Autodesk Inventor part; units mm, degrees
ref_plane "YZ Plane" through (0, 0, 0) normal (1, 0, 0) x (0, 1, 0)
ref_plane "XZ Plane" through (0, 0, 0) normal (0, 1, 0) x (-1, 0, 0)
ref_plane "XY Plane" through (0, 0, 0) normal (0, 0, 1) x (1, 0, 0)
sketch "Sketch1" plane through (0, 0, 0) normal (0, 0, 1) x (1, 0, 0)
  line L0 (-22, -22) -> (22, -22)
  line L1 (22, -22) -> (22, 22)
  line L2 (22, 22) -> (-22, 22)
  line L3 (-22, 22) -> (-22, -22)
  line L4 (-22, -22) -> (22, 22) construction
  line L5 (22, -22) -> (-22, 22) construction
  point P0 (0, 0)
  point P1 (0, 0)
  dimension "a" = 44
  dimension "d10" = 22
  dimension "d11" = 22
  dimension "d15" = 44
extrude "Extrusion1" add sketch "Sketch1" along normal blind 10
sketch "Sketch2" plane through (0, 0, 10) normal (0, 0, 1) x (1, 0, 0)
  circle A0 centre (0, 0) radius 18
  dimension "dg6" = 36
extrude "Extrusion2" add sketch "Sketch2" along normal blind 17
sketch "Sketch3" plane through (0, 0, 27) normal (0, 0, 1) x (1, 0, 0)
  circle A0 centre (0, 0) radius 18
  circle A1 centre (0, 0) radius 6
  dimension "d1" = 12
extrude "Extrusion3" cut sketch "Sketch3" against normal through all contours A1
chamfer "Chamfer1" distance 5 angle 45 4 edges at (22, 22, 5) (22, -22, 5) (-22, -22, 5) (-22, 22, 5)
sketch "Sketch4" plane through (0, 0, 0) normal (0, 0, -1) x (-1, 0, 0)
  circle A0 centre (0, 0) radius 6
  circle A1 centre (0, 0) radius 22 construction
  point P0 (17, 13.9642)
  point P1 (-17, -13.9642)
  point P2 (-17, 13.9642)
  point P3 (17, -13.9642)
  dimension "d16" = 44
  dimension "d17" = 34
hole "Hole1" at (-17, 13.9642, 0) at (17, -13.9642, 0) at (17, 13.9642, 0) at (-17, -13.9642, 0) direction (0, 0, 1) diameter 4.5 end through all
sketch "Sketch5" plane through (0, 0, 0) normal (0, 0, -1) x (-1, 0, 0)
  circle A0 centre (-17, 13.9642) radius 2.25
  circle A1 centre (17, 13.9642) radius 2.25
  circle A2 centre (-17, -13.9642) radius 2.25
  circle A3 centre (17, -13.9642) radius 2.25
hole "Hole2" at (17, 13.9642, 0) at (-17, 13.9642, 0) at (-17, -13.9642, 0) at (17, -13.9642, 0) direction (0, 0, 1) diameter 8 depth 4
equation "\"d15\" = a"
properties part number "fk12"
Verification items for the finished model (mm, model axes). A direction names the side the tool comes from. Coordinates: 2 decimals unless noted, no trailing zeros. Loops run counter-clockwise (first coordinate to the right, second up) from the corner with the lowest first, then second, coordinate; pieces in that order, holes last. Notation, with made-up numbers: (71, 37) -> (107, 37) arc R15 cw to (107, 46) -> close; hole circle Ø5 at (65, 73). An arc over 180 degrees is marked (long way). Answer in a Markdown table with one row per item.
1) Section check C-C (z = 17.5). Record the cut outline in (x, y).
The answers:
| item | result |
|---|---|
| outline | circle Ø36 at (0, 0); hole circle Ø12 at (0, 0) |
2) Access from +Z, -Z, +X, -X, +Y, -Y to the whole of each face (thin tool, end or side, straight path). Record for faces 1 (the face through (-15, -12, 4)), 2 (the face through (0, 20, 10)), 3 (the face through (-19, -20, 5)).
The answers:
| item | result |
|---|---|
| face 1 | -Z |
| face 2 | +Z |
| face 3 | +Z, -Z, -X, -Y |
3) Scan lines: line 1 along Y through (x, z) = (-17, 7); line 2 along Y through (x, z) = (-17, 1.25); line 3 along Y through (x, z) = (0, 18). Record each from-to range of solid material in increasing order. Write a range as from..to.
The answers:
| item | result |
|---|---|
| line 1 | y = -22..-16.21, -11.71..11.71, 16.21..22 |
| line 2 | y = -22..-17.96, -9.96..9.96, 17.96..22 |
| line 3 | y = -18..-6, 6..18 |
4) Depth check by flat-ended pin: P1, Ø6, axis at x = 17, y = 13.96, coming from the +Z side; P2, Ø2, axis at y = -15, z = 16.5, coming from the +X side; P3, Ø6, axis at x = -4, z = 22, coming from the -Y side. Enter the tip coordinate at first touch or a pass-through.
The answers:
| item | result |
|---|---|
| P1 | stops at z = 10 |
| P2 | stops at x = 11.31 |
| P3 | stops at y = -17.97 |
5) Draft check along X on faces 4 (the face through (5, -5, 0)), 5 (the face through (19, 16, 4)), 6 (the face through (20, 19, 5)). Enter one of: released by +X, released by -X, zero draft, split by the parting line, or undercut.
The answers:
| item | result |
|---|---|
| face 4 | zero draft |
| face 5 | undercut |
| face 6 | released by +X |
6) Section check A-A (x = 0). Record the cut outline in (y, z), and give its area (3 significant figures).
The answers:
| item | result |
|---|---|
| outline | (-22, 0) -> (-6, 0) -> (-6, 27) -> (-18, 27) -> (-18, 10) -> (-22, 10) -> close; (6, 0) -> (22, 0) -> (22, 10) -> (18, 10) -> (18, 27) -> (6, 27) -> close |
| area | 728 mm2 |
7) Section check D-D (y = 9). Record the cut outline in (x, z).
The answers:
| item | result |
|---|---|
| outline | (-22, 0) -> (22, 0) -> (22, 10) -> (15.59, 10) -> (15.59, 27) -> (-15.59, 27) -> (-15.59, 10) -> (-22, 10) -> close |
